Geometry: final body of the model. Coordinates: model frame, mm. Give positions to 0.01 mm unless a question says otherwise; leave off trailing zeros. Write each loop counter-clockwise with the first axis right and the second up, starting at its lowest first coordinate (ties: lowest second). Pieces come first, ordered by that corner, then holes. Notation, with made-up numbers: (28.5, -34) -> (65.5, -34) arc R20 cw to (65.5, 3) -> close; hole circle Ø6 at (47, 71). An arc over 180 degrees is marked (long way). Answer as a JSON object with one key per item and string values.
from build123d import *

# Parameters (mm, degrees)
F1_DEPTH = 25.4
F3_DEPTH = 914.4
F4_R     = 6.35
F6_DEPTH = 914.401


with BuildPart() as f1:
    # F0 (on Front) → F1 (new body)
    with BuildSketch(Plane.XZ):
        Polygon((483.0016511798, 164.7552716235), (-431.3983488202, 164.7552716235), (-431.3983488202, -292.4447283765), (-380.5983488202, -292.4447283765), (-380.5983488202, -154.1671283765), (-355.1983488202, -154.1671283765), (-355.1983488202, -292.4447283765), (406.8016511798, -292.4447283765), (406.8016511798, -154.1671283765), (432.2016511798, -154.1671283765), (432.2016511798, -292.4447283765), (483.0016511798, -292.4447283765), align=None)
    extrude(amount=F1_DEPTH)

    # F2 (on face) → F3 (cut)
    with BuildSketch(Plane.YZ.offset(483.0016511798)):
        Polygon((0, 164.7552716235), (-25.4, 164.7552716235), (0, 160.2765663135), align=None)
    extrude(amount=-F3_DEPTH, mode=Mode.SUBTRACT)

    # F4
    f4_edges = [f1.edges().sort_by_distance(p)[0] for p in [
        (25.801651, 0, 160.276566),
        (25.801651, -25.4, 164.755272),
    ]]
    fillet(f4_edges, radius=F4_R)

    # F5 (on face) → F6 (cut, through all)
    with BuildSketch(Plane.YZ.offset(483.0016511798)):
        Polygon((-25.4, -292.4447283765), (0, -292.4447283765), (-25.4, -285.6388188887), align=None)
    extrude(amount=-F6_DEPTH, mode=Mode.SUBTRACT)


solid = f1.part
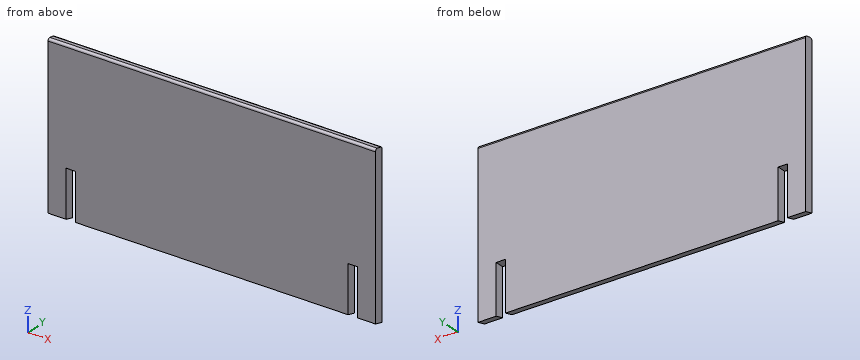
Q1. First-contact query: P1, Ø10, axis at x = 4, y = -7, coming from the +Z side; P2, Ø12.5, axis at x = 423.5, y = -12, coming from the -Z side. Flat tips, straight axial feed; report the tip coordinate or a pass-through.
Values:
{"P1": "z = 162.39", "P2": "z = -154.17"}
Q2. Cut plane A-A (z = -232). Return the cut outline in (x, y), and give its area (3 significant figures).
Values:
{"outline": "(-431.4, -25.4) -> (-380.6, -25.4) -> (-380.6, 0) -> (-431.4, 0) -> close; (-355.2, -25.4) -> (406.8, -25.4) -> (406.8, 0) -> (-355.2, 0) -> close; (432.2, -25.4) -> (483, -25.4) -> (483, 0) -> (432.2, 0) -> close", "area": "21,900 mm²"}
Q3. Cut plane B-B (y = -14). Return the cut outline in (x, z), and give its area (3 significant figures).
Values:
{"outline": "(-431.4, -288.69) -> (-380.6, -288.69) -> (-380.6, -154.17) -> (-355.2, -154.17) -> (-355.2, -288.69) -> (406.8, -288.69) -> (406.8, -154.17) -> (432.2, -154.17) -> (432.2, -288.69) -> (483, -288.69) -> (483, 162.75) -> (-431.4, 162.75) -> close", "area": "406,000 mm²"}
Q4. Material intervals for L1, parallel to X at y = -17.25, z = -230; L2, parallel to Z at x = -266.5, y = -19.5; L3, parallel to Z at x = 300, y = -8, sorted ascending. Write a range as from..to.
Values:
{"L1": "-431.4..-380.6, -355.2..406.8, 432.2..483", "L2": "-287.22..163.52", "L3": "-290.3..161.69"}
